Build history of the part. All positions in model axes, mm. Coordinates: 2 decimals unless noted, no trailing zeros. Order: outer loops, then holes, each group sorted by start corner. A loop starts at its lowest first (then second) coordinate and runs counter-clockwise, first axis right, second up. Notation, with made-up numbers: (62, 35) - (76, 35) arc R25 cw to (76, 51) - close; hole circle Ø5 at (60, -34). An arc over 180 degrees is marked (long way). Write each question's results on one line, items separated by ' | '. Start each with the question number.
from build123d import *

# Parameters (mm, degrees)
F0_W     = 1400
F0_H     = 2300
F1_DEPTH = 50
F2_SIZE2 = 49.99999
F2_SIZE  = 29.99999


# Not quite as in the source:
# - a fillet or chamfer is up to 0.001 mm smaller than in the source, because OpenCascade refuses the exact size


with BuildPart() as f1:
    # F0 (on Top) → F1 (new body)
    with BuildSketch(Plane.XY):
        Rectangle(F0_W, F0_H)
    extrude(amount=F1_DEPTH)

    # F2 (size 30 and 50 in the source; OpenCascade refuses exactly that, so slightly less here)
    f2_edges = [f1.edges().sort_by_distance(p)[0] for p in [
        (0, -1150, 50),
        (700, 0, 50),
        (0, 1150, 50),
        (-700, 0, 50),
    ]]
    f2_side = f1.faces().sort_by_distance((0, 0, 50))[0]
    chamfer(f2_edges, length=F2_SIZE, length2=F2_SIZE2, reference=f2_side)


solid = f1.part
Item 1: Probe probe 1 along X at (y, z) = (980, 3); probe 2 along Y at (x, z) = (330, 38.5); probe 3 along X at (y, z) = (817, 23). List the from-to ranges inside material, lowest first.
Item 2: Flat gauge pins, fed straight in: P1, Ø8, axis at x = -540, z = 37.5, coming from the +Y side; P2, Ø8, axis at y = 352, z = 15, coming from the -X side; P3, Ø3, axis at x = 172.5, z = 8.5, coming from the +Y side; P4, Ø8, axis at x = 403.5, y = 362, coming from the -Z side. Where does each tip first touch, or does it go through?
Item 3: Pull direction Z, two halves, no side cores. Call faces 1 (the flat face through (-10, 16, 0)), 2 (the flat face through (-10, 1135, 25)): released by +Z, released by -Z, zero draft, split by the parting line, or undercut.
Item 4: Slice it at B-B (z = 36). Write the cut outline in (x, y), then the cut area to 3 significant figures.
Resolved:
1) probe 1: -698.2 to 698.2 | probe 2: -1126.9 to 1126.9 | probe 3: -686.2 to 686.2
2) P1: y = 1129.9 | P2: x = -693.4 | P3: y = 1145.8 | P4: z = 0
3) face 1: released by -Z | face 2: released by +Z
4) outline: (-678.4, -1128.4) - (678.4, -1128.4) - (678.4, 1128.4) - (-678.4, 1128.4) - close | area: 3,060,000 mm^2
